Could you check a few things on this drawing? It's one solid part, dimensions in mm from its lowest x, y, z. Round coordinates to 2 decimals unless told otherwise and drop trailing zeros. Order: outer loops, then holes, each group sorted by start corner. A loop starts at its lowest first (then second) coordinate and runs counter-clockwise, first axis right, second up. Notation, with made-up numbers: (-21, 45.5) - (-7, 45.5) arc R34 cw to (-7, 84.5) - close; hole circle Ø11 at (-5.5, 11.25). An arc over 180 degrees is marked (long way). Use one line per item in the form item = value.
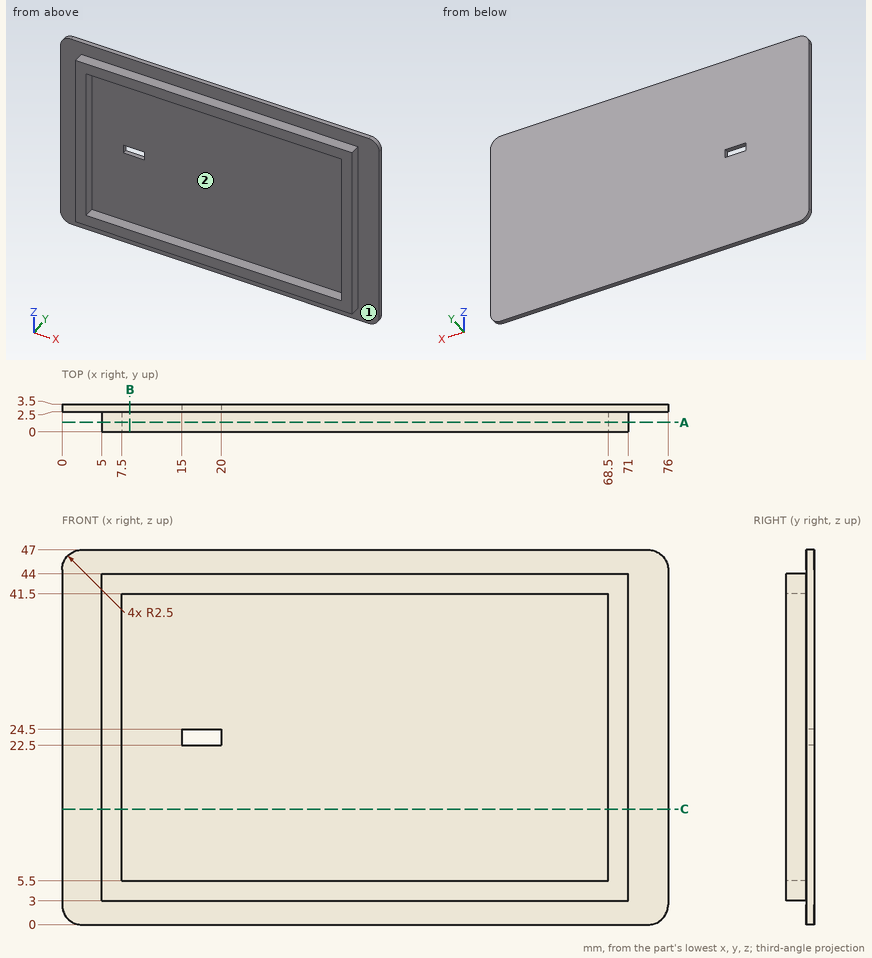
Item 1: If we mould it in two halves opening along X, with no side actions, what happens to the marked faces 1 and 2? For each: released by +X, released by -X, zero draft, split by the parting line, or undercut.
Found:
face_1 = zero draft
face_2 = undercut
Item 2: Imagine slicing it at C-C on z = 14.5. Please give me the cut outline in (x, y), plus the area to 3 significant figures.
Found:
outline = (0, 2.5) - (5, 2.5) - (5, 0) - (7.5, 0) - (7.5, 2.5) - (68.5, 2.5) - (68.5, 0) - (71, 0) - (71, 2.5) - (76, 2.5) - (76, 3.5) - (0, 3.5) - close
area = 88.5 mm2
Item 3: Imagine slicing it at B-B on x = 8.5. Please give me the cut outline in (y, z).
Found:
outline = (0, 3) - (2.5, 3) - (2.5, 0) - (3.5, 0) - (3.5, 47) - (2.5, 47) - (2.5, 44) - (0, 44) - (0, 41.5) - (2.5, 41.5) - (2.5, 5.5) - (0, 5.5) - close
Item 4: Will these pins go through, and if not, where does the flat tip stop? P1, Ø14, axis at x = 46, z = 15.5, coming from the -Y side; P2, Ø0.8, axis at y = 1, z = 16, coming from the -X side; P3, Ø0.8, axis at x = 38.5, y = 1.5, coming from the -Z side.
Found:
P1 = 2.5
P2 = 5
P3 = 3
Item 5: I need wall thicknesses on L1, parallel to Z at x = 47.5, y = 2.2; L2, parallel to Z at x = 16, y = 2.9; L3, parallel to X at y = 0.85, z = 16. Which ranges of each line are inside material? Lowest first, please.
Found:
L1 = 3 to 5.5, 41.5 to 44
L2 = 0 to 22.5, 24.5 to 47
L3 = 5 to 7.5, 68.5 to 71
Item 6: Imagine slicing it at A-A on y = 1.2. Please give me the cut outline in (x, z).
Found:
outline = (5, 3) - (71, 3) - (71, 44) - (5, 44) - close; hole (7.5, 5.5) - (68.5, 5.5) - (68.5, 41.5) - (7.5, 41.5) - close
